```python
from build123d import *

# Parameters (mm, degrees)
SKETCH4_R           = 4
BOSS_EXTRUDE1_DEPTH = 40
SKETCH5_R           = 1.75
CUT_EXTRUDE1_DEPTH  = 15
SKETCH6_W           = 59.399220689
SKETCH6_H           = 23.559499922
CUT_EXTRUDE3_DEPTH  = 30
BOSS_EXTRUDE2_DEPTH = 40


with BuildPart() as part:
    # Sketch4 → Boss-Extrude1 (new body)
    # profile 1 of 2: a face of its own
    with BuildSketch(Plane.XY):
        Polygon((0, -45), (37.5, -45), (37.5, 15.206160185), (12.5, 45), (0, 45), align=None)
        with Locations((14.5, -14.279076444)):
            Circle(SKETCH4_R, mode=Mode.SUBTRACT)
        with Locations((22.5, 14.634588146)):
            Circle(SKETCH4_R, mode=Mode.SUBTRACT)
        with Locations((8, 35)):
            Circle(SKETCH4_R, mode=Mode.SUBTRACT)
    # profile 2 of 2: a face of its own
    with BuildSketch(Plane.XY):
        Polygon((-37.5, -45), (0, -45), (0, 45), (-12.5, 45), (-37.5, 15.206160185), align=None)
        with Locations((-22.5, 14.634588146)):
            Circle(SKETCH4_R, mode=Mode.SUBTRACT)
        with Locations((-8, 35)):
            Circle(SKETCH4_R, mode=Mode.SUBTRACT)
    extrude(amount=BOSS_EXTRUDE1_DEPTH)

    # Sketch5 → Cut-Extrude1 (cut)
    with BuildSketch(Plane.XZ.offset(45)):
        with Locations((-30, 7.15)):
            Circle(SKETCH5_R)
        with Locations(Location((30, 7.15, 0), (0, 0, 180))):
            Circle(SKETCH5_R)
        with Locations((30, 32.85)):
            Circle(SKETCH5_R)
        with Locations(Location((-30, 32.85, 0), (0, 0, 180))):
            Circle(SKETCH5_R)
    extrude(amount=-CUT_EXTRUDE1_DEPTH, mode=Mode.SUBTRACT)

    # Sketch6 → Cut-Extrude3 (cut)
    with BuildSketch(Plane(origin=(0, 0, 0), x_dir=(-1, 0, 0), z_dir=(0, 0, -1))):
        with Locations((-4.650193569, -14.217324683)):
            Rectangle(SKETCH6_W, SKETCH6_H)
    extrude(amount=-CUT_EXTRUDE3_DEPTH, mode=Mode.SUBTRACT)

    # Sketch7 → Boss-Extrude2 (add)
    with BuildSketch(Plane.XY.offset(40)):
        Polygon((-37.5, 15.206160185), (-55.5, -45), (-37.5, -45), align=None)
        Polygon((37.5, -45), (37.5, 15.206160185), (55.5, -45), align=None)
    extrude(amount=-BOSS_EXTRUDE2_DEPTH)


solid = part.part
```
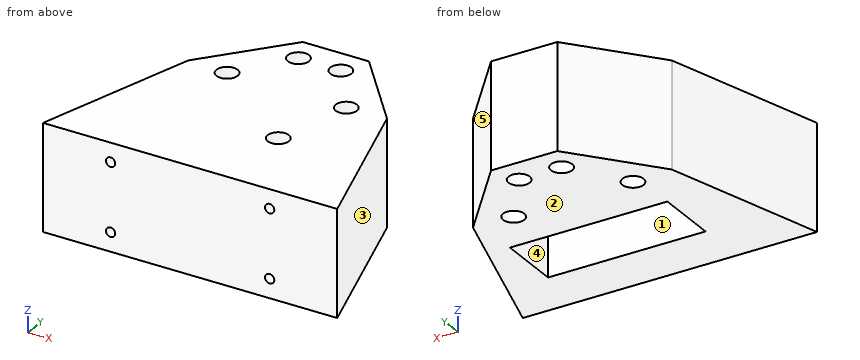
Model file for the job. Use its own axes, mm. Face numbers are marked on the shaded views. A direction names the side the tool comes from. Coordinates: 2 decimals unless noted, no trailing zeros. Loops run counter-clockwise (first coordinate to the right, second up) from the corner with the lowest first, then second, coordinate; pieces in that order, holes last. Notation, with made-up numbers: (46, 15.5) -> (99, 15.5) arc R35 cw to (99, 54.5) -> close; hole circle Ø2 at (55, 60.5). An arc over 180 degrees is marked (long way). Answer as a JSON object with one key per item and string values.
Q1. Cut at C-C (z = 32.85). List the corners of the cut face in (x, y).
Report:
{"outline": "(-55.5, -45) -> (-31.75, -45) -> (-31.75, -30) -> (-28.25, -30) -> (-28.25, -45) -> (28.25, -45) -> (28.25, -30) -> (31.75, -30) -> (31.75, -45) -> (55.5, -45) -> (37.5, 15.21) -> (12.5, 45) -> (-12.5, 45) -> (-37.5, 15.21) -> close; hole circle Ø8 at (-22.5, 14.63); hole circle Ø8 at (-8, 35); hole circle Ø8 at (8, 35); hole circle Ø8 at (14.5, -14.28); hole circle Ø8 at (22.5, 14.63)"}
Q2. Cut at D-D (x = 22). List the corners of the cut face in (y, z), and give its area (3 significant figures).
Report:
{"outline": "(-45, 0) -> (-26, 0) -> (-26, 30) -> (-2.44, 30) -> (-2.44, 0) -> (10.67, 0) -> (10.67, 40) -> (-45, 40) -> close; (18.6, 0) -> (33.68, 0) -> (33.68, 40) -> (18.6, 40) -> close", "area": "2,120 mm2"}
Q3. Cut at B-B (y = 35). List the corners of the cut face in (x, z), and give its area (3 significant figures).
Report:
{"outline": "(-20.89, 0) -> (-12, 0) -> (-12, 40) -> (-20.89, 40) -> close; (-4, 0) -> (4, 0) -> (4, 40) -> (-4, 40) -> close; (12, 0) -> (20.89, 0) -> (20.89, 40) -> (12, 40) -> close", "area": "1,030 mm2"}
Q4. Flat gauge pins, fed straight in: P1, Ø1, axis at x = -29.5, z = 32.5, coming from the -Y side; P2, Ø12, axis at y = -12.5, z = 22, coming from the +X side; P3, Ø10, axis at y = -6.5, z = 36, coming from the -X side. Where does each tip first touch, or does it go through?
Report:
{"P1": "stops at y = -30", "P2": "stops at x = 47.58", "P3": "stops at x = -45.48"}
Q5. 3-axis set-ups, long thin cutter, end or side, ignore diameter. For the marked faces 4 and 5: which of +Z, -Z, +X, -X, +Y, -Y reach the whole face in a straight line?
Report:
{"face 4": "-Z", "face 5": "+Z, -Z, +X, +Y"}
Q6. Probe probe 1 along Z at (x, y) = (-30, -40); probe 2 along Y at (x, z) = (8, 10); probe 3 along Y at (x, z) = (12.5, 9). List the from-to ranges inside material, lowest first.
Report:
{"probe 1": "z = 0 to 5.4, 8.9 to 31.1, 34.6 to 40", "probe 2": "y = -45 to -26, -2.44 to 31, 39 to 45", "probe 3": "y = -45 to -26, -2.44 to 45"}
Q7. Pull direction Y, two halves, no side cores. Call the marked faces 1, 2 and 3: released by +Y, released by -Y, zero draft, split by the parting line, or undercut.
Report:
{"face 1": "undercut", "face 2": "zero draft", "face 3": "released by +Y"}
Q8. Cut at A-A (x = -8). List the corners of the cut face in (y, z).
Report:
{"outline": "(-45, 0) -> (-26, 0) -> (-26, 30) -> (-2.44, 30) -> (-2.44, 0) -> (31, 0) -> (31, 40) -> (-45, 40) -> close; (39, 0) -> (45, 0) -> (45, 40) -> (39, 40) -> close"}
